The model under review builds one solid part; all positions refer to its coordinate system, in mm. Face numbers are marked on the shaded views. A direction names the side the tool comes from. Coordinates: 2 decimals unless noted, no trailing zeros. Loops run counter-clockwise (first coordinate to the right, second up) from the corner with the lowest first, then second, coordinate; pieces in that order, holes last. Notation, with made-up numbers: (46.5, 18.25) - (105.5, 18.25) arc R21 cw to (105.5, 43.25) - close; hole circle Ø4 at (10.5, -5). An arc over 180 degrees is marked (long way). One line per item, written item: value. Start each with the question number.
1. We need section A-A, the plane x = 10. Give the boundary of the cut face in (y, z), then the cut area to 3 significant figures.
2. We need section B-B, the plane z = 10. Give the boundary of the cut face in (x, y), then the cut area to 3 significant figures.
3. To check wall thickness, follow line 1 (X direction, y = 37.7, z = 35); line 2 (X direction, y = 24, z = 35.5). State the ranges of each line that lie inside material, in increasing order.
4. We need section C-C, the plane y = 12. Give the boundary of the cut face in (x, z), then the cut area to 3 significant figures.
5. Insertion check: P1, Ø4, axis at x = 4.5, y = 27, coming from the +Z side; P2, Ø12, axis at x = 19, y = 27, coming from the +Z side; P3, Ø1.5, axis at y = 38.5, z = 8.5, coming from the -X side; P4, Ø2, axis at x = 35, z = 5, coming from the +Y side. Each pin has a flat end and moves straight along its axis. Give the tip position at first contact, or say it passes through.
6. For the marked faces 1 and 2, list the 3-axis set-ups (+Z, -Z, +X, -X, +Y, -Y) from which the entire face can be reached by the end or side of a thin tool; tool diameter is ignored.
7. Mouldability with a two-part tool opening along X and no side actions: class the marked faces 3, 4, 5 and 6 as +X half, -X half, draft (parallel to the pull), parting line (faces both ways), or undercut.
8. We need section D-D, the plane y = 20. Give the boundary of the cut face in (x, z).
Autodesk Inventor part; units mm, degrees
ref_plane "YZ Plane" through (0, 0, 0) normal (1, 0, 0) x (0, 1, 0)
ref_plane "XZ Plane" through (0, 0, 0) normal (0, 1, 0) x (-1, 0, 0)
ref_plane "XY Plane" through (0, 0, 0) normal (0, 0, 1) x (1, 0, 0)
sketch "スケッチ1" plane through (0, 0, 0) normal (0, 0, 1) x (1, 0, 0)
  line L0 (0, 0) -> (40, 0)
  line L1 (40, 0) -> (40, 40)
  line L2 (40, 40) -> (0, 40)
  line L3 (0, 40) -> (0, 0)
  dimension "d0" = 40
  dimension "d1" = 40
extrude "押し出し1" add sketch "スケッチ1" along normal blind 40
shell "シェル1" thickness 3 removed faces 2 at (26.6667, 13.3333, 0) at (26.6667, 13.3333, 40)
sketch "スケッチ2" plane through (0, 0, 0) normal (-1, 0, 0) x (0, 0, 1)
  line L0 (0, 40) -> (0, 0)
  line L1 (0, 40) -> (40, 40)
  line L2 (0, 0) -> (27, 0)
  line L3 (27, 0) -> (27, 40)
  line L4 (27, 40) -> (0, 40)
  line L5 (0, 40) -> (0, 0)
  dimension "d5" = 27
extrude "押し出し2" cut sketch "スケッチ2" against normal blind 5
sketch "スケッチ3" plane through (0, 0, 40) normal (-1, 0, 0) x (0, 0, 1)
  circle A0 centre (-7, 20) radius 1.5
  line L0 (0, 40) -> (0, 0)
  line L1 (-13, 0) -> (0, 0)
  point P0 (-40, 0)
  dimension "d8" = 3
  dimension "d9" = 7
  dimension "d10" = 20
hole "穴1" at (0, 20, 33) direction (1, 0, 0) diameter 3 end through all
sketch "スケッチ4" plane through (0, 40, 40) normal (0, 1, 0) x (1, 0, 0)
  line L0 (35, 35) -> (10, 35)
  line L1 (10, 35) -> (10, 5)
  line L2 (10, 5) -> (35, 5)
  line L3 (35, 5) -> (35, 35)
  line L4 (40, 40) -> (5, 40)
  line L5 (40, 40) -> (40, 0)
  point P0 (0, 40)
  dimension "d18" = 25
  dimension "d19" = 30
  dimension "d20" = 5
  dimension "d21" = 5
hole "穴2" at (10, 40, 5) at (35, 40, 5) at (35, 40, 35) at (10, 40, 35) direction (0, -1, 0) diameter 2.459 depth 3
sketch "スケッチ5" plane through (40, 0, 0) normal (1, 0, 0) x (0, 0, -1)
  line L0 (0, 0) -> (-40, 0)
  line L1 (0, 0) -> (0, 40)
  point P0 (-10, 12)
  point P1 (-10, 28)
  dimension "d29" = 16
  dimension "d32" = 12
  dimension "d33" = 10
  dimension "d34" = 10
hole "穴3" at (40, 28, 10) at (40, 12, 10) direction (-1, 0, 0) diameter 2.8 depth 3
sketch "スケッチ6" plane through (40, 0, 0) normal (1, 0, 0) x (0, 0, -1)
  circle A0 centre (-10, 20) radius 5
  line L0 (0, 0) -> (0, 40)
  line L1 (0, 0) -> (-40, 0)
  dimension "d42" = 10
  dimension "d43" = 10
  dimension "d44" = 20
extrude "押し出し3" cut sketch "スケッチ6" against normal blind 5
properties part number "ギヤボックス２右"
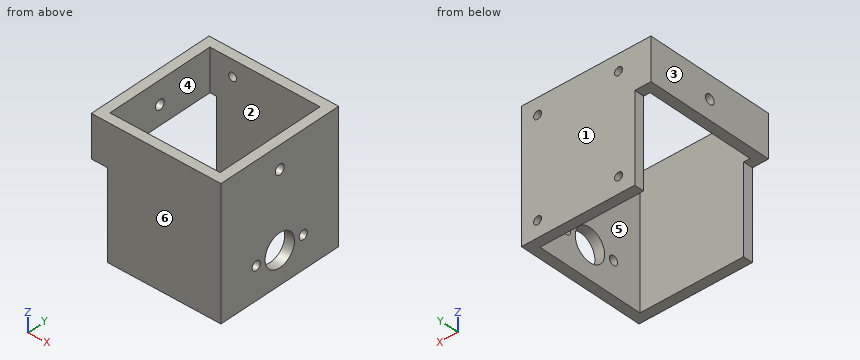
Findings below:
1. outline: (0, 0) - (3, 0) - (3, 40) - (0, 40) - close; (37, 0) - (40, 0) - (40, 3.77) - (37, 3.77) - close; (37, 6.23) - (40, 6.23) - (40, 33.77) - (37, 33.77) - close; (37, 36.23) - (40, 36.23) - (40, 40) - (37, 40) - close
1. area: 225 mm2
2. outline: (5, 0) - (40, 0) - (40, 10.6) - (37, 10.6) - (37, 3) - (5, 3) - close; (5, 37) - (37, 37) - (37, 29.4) - (40, 29.4) - (40, 40) - (5, 40) - close; (37, 13.4) - (40, 13.4) - (40, 15) - (37, 15) - close; (37, 25) - (40, 25) - (40, 26.6) - (37, 26.6) - close
2. area: 265 mm2
3. line 1: 0 to 8.77, 11.23 to 33.77, 36.23 to 40
3. line 2: 0 to 3, 37 to 40
4. outline: (0, 27) - (3, 27) - (3, 40) - (0, 40) - close; (37, 0) - (40, 0) - (40, 8.6) - (37, 8.6) - close; (37, 11.4) - (40, 11.4) - (40, 40) - (37, 40) - close
4. area: 151 mm2
5. P1: z = 40
5. P2: through
5. P3: x = 5
5. P4: y = 3
6. face 1: +Z, -Z, +X, -X, +Y
6. face 2: +Z, -Z
7. face 3: -X half
7. face 4: undercut
7. face 5: undercut
7. face 6: draft
8. outline: (0, 27) - (3, 27) - (3, 31.5) - (0, 31.5) - close; (0, 34.5) - (3, 34.5) - (3, 40) - (0, 40) - close; (37, 0) - (40, 0) - (40, 5) - (37, 5) - close; (37, 15) - (40, 15) - (40, 31.5) - (37, 31.5) - close; (37, 34.5) - (40, 34.5) - (40, 40) - (37, 40) - close
